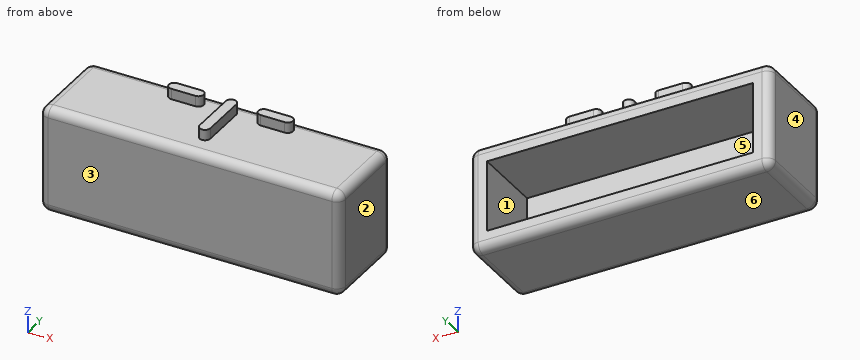
```python
from build123d import *

# Parameters (mm, degrees)
SKETCH_1_W          = 75
SKETCH_1_H          = 20
EXTRUDE_1_DEPTH     = 20
SKETCH_2_W          = 85
SKETCH_2_H          = 30
EXTRUDE_2_DEPTH     = 25
SKETCH_3_W          = 75
SKETCH_3_H          = 20
CUT_EXTRUDE_1_DEPTH = 20
EXTRUDE_3_DEPTH     = 3
FILLET_1_R          = 2.5


with BuildPart() as part:
    # Sketch 1 → Extrude 1 (new body)
    with BuildSketch(Plane(origin=(0, 0, 0), x_dir=(1, 0, 0), z_dir=(0, 1, 0))):
        Rectangle(SKETCH_1_W, SKETCH_1_H)
    extrude(amount=-EXTRUDE_1_DEPTH)

    # Sketch 2 → Extrude 2 (add)
    with BuildSketch(Plane(origin=(0, 0, 0), x_dir=(1, 0, 0), z_dir=(0, 1, 0))):
        Rectangle(SKETCH_2_W, SKETCH_2_H)
    extrude(amount=-EXTRUDE_2_DEPTH)

    # Sketch 3 → Cut-Extrude 1 (cut)
    with BuildSketch(Plane(origin=(0, 0, 0), x_dir=(1, 0, 0), z_dir=(0, 1, 0))):
        Rectangle(SKETCH_3_W, SKETCH_3_H)
    extrude(amount=-CUT_EXTRUDE_1_DEPTH, mode=Mode.SUBTRACT)

    # Sketch 5 → Extrude 3 (add)
    with BuildSketch(Plane.XY.offset(15)):
        with BuildLine():
            Line((-16, -3), (-9.2, -3))
            ThreePointArc((-9.2, -3), (-7.7, -4.5), (-9.2, -6))
            Line((-9.2, -6), (-16, -6))
            ThreePointArc((-16, -6), (-17.5, -4.5), (-16, -3))
        make_face()
        with BuildLine():
            Line((16, -3), (9.2, -3))
            ThreePointArc((9.2, -3), (7.7, -4.5), (9.2, -6))
            Line((9.2, -6), (16, -6))
            ThreePointArc((16, -6), (17.5, -4.5), (16, -3))
        make_face()
        with BuildLine():
            Line((1.5, -4.5), (1.5, -17.5))
            ThreePointArc((1.5, -17.5), (0, -19), (-1.5, -17.5))
            Line((-1.5, -17.5), (-1.5, -4.5))
            ThreePointArc((-1.5, -4.5), (0, -3), (1.5, -4.5))
        make_face()
    extrude(amount=EXTRUDE_3_DEPTH)

    # Fillet 1
    fillet_1_edges = [part.edges().sort_by_distance(p)[0] for p in [
        (0, -25, -15),
        (-42.5, -12.5, -15),
        (42.5, -25, 0),
        (42.5, -12.5, -15),
        (0, -25, 15),
        (42.5, -12.5, 15),
        (-42.5, -25, 0),
        (-42.5, -12.5, 15),
        (0, 0, -15),
        (-42.5, 0, 0),
        (0, 0, 15),
        (42.5, 0, 0),
    ]]
    fillet(fillet_1_edges, radius=FILLET_1_R)


solid = part.part
```
CAD build for the part. Positions are in the model's coordinates, mm. Face numbers are marked on the shaded views. A direction names the side the tool comes from. Round coordinates to 2 decimals unless told otherwise and drop trailing zeros. Order: outer loops, then holes, each group sorted by start corner. A loop starts at its lowest first (then second) coordinate and runs counter-clockwise, first axis right, second up. Notation, with made-up numbers: (76, -21) - (81, -21) arc R11 cw to (81, -12) - close; hole circle Ø11 at (-13, 52). An arc over 180 degrees is marked (long way). Answer in a Markdown table with one row per item. Add a question column.
(1) Band-saw the part on A-A on z = -9. List the corners of the cut face in (x, y).
(2) Mould opens along X. For the marked faces 1, 2, 3 and 4 say: +X half, -X half, draft (parallel to the pull), parting line (faces both ways), or undercut.
(3) Band-saw the part on C-C on y = -14.5. List the corners of the cut face in (x, z), and give its area (3 significant figures).
(4) Band-saw the part on B-B on x = 25. List the corners of the cut face in (y, z), and give its area (3 significant figures).
(5) Probe L1, parallel to Z at x = 7.5, y = -19; L2, parallel to X at y = -9, z = 4; L3, parallel to Z at x = 13, y = -4.75. List the from-to ranges inside material, lowest first. Write a range as [from, to].
(6) Drop flat-ended pins along their axis: pin 1 Ø2.5 at (x, z) = (13, 16) entering from -Y; pin 2 Ø1.5 at (x, z) = (-12.5, 16) entering from +Y; pin 3 Ø5 at (x, y) = (-22, -12) entering from +Z. Give the stop position or say it passes through.
(7) 3-axis set-ups, long thin cutter, end or side, ignore diameter. For the marked faces 5 and 6: which of +Z, -Z, +X, -X, +Y, -Y reach the whole face in a straight line?
Data:
| question | item | result |
|---|---|---|
| 1 | outline | (-42.5, -22.5) arc R2.5 ccw to (-40, -25) - (40, -25) arc R2.5 ccw to (42.5, -22.5) - (42.5, -2.5) arc R2.5 ccw to (40, 0) - (37.5, 0) - (37.5, -20) - (-37.5, -20) - (-37.5, 0) - (-40, 0) arc R2.5 ccw to (-42.5, -2.5) - close |
| 2 | face 1 | undercut |
| 2 | face 2 | +X half |
| 2 | face 3 | draft |
| 2 | face 4 | -X half |
| 3 | outline | (-42.5, -12.5) arc R2.5 ccw to (-40, -15) - (40, -15) arc R2.5 ccw to (42.5, -12.5) - (42.5, 12.5) arc R2.5 ccw to (40, 15) - (1.5, 15) - (1.5, 18) - (-1.5, 18) - (-1.5, 15) - (-40, 15) arc R2.5 ccw to (-42.5, 12.5) - close; hole (-37.5, -10) - (37.5, -10) - (37.5, 10) - (-37.5, 10) - close |
| 3 | area | 1,050 mm^2 |
| 4 | outline | (-25, -12.5) arc R2.5 ccw to (-22.5, -15) - (-2.5, -15) arc R2.5 ccw to (0, -12.5) - (0, -10) - (-20, -10) - (-20, 10) - (0, 10) - (0, 12.5) arc R2.5 ccw to (-2.5, 15) - (-22.5, 15) arc R2.5 ccw to (-25, 12.5) - close |
| 4 | area | 345 mm^2 |
| 5 | L1 | z = [-15, -10], [10, 15] |
| 5 | L2 | x = [-42.5, -37.5], [37.5, 42.5] |
| 5 | L3 | z = [-15, -10], [10, 18] |
| 6 | pin 1 | stops at y = -23.59 |
| 6 | pin 2 | stops at y = -3 |
| 6 | pin 3 | stops at z = 15 |
| 7 | face 5 | +Y |
| 7 | face 6 | -Z, +X, -X, +Y, -Y |
